The drawing under review shows one solid part. Ordinate dimensions are in mm from its lowest x, y, z. A direction names the side the tool comes from. Round coordinates to 2 decimals unless told otherwise and drop trailing zeros. Order: outer loops, then holes, each group sorted by start corner. A loop starts at its lowest first (then second) coordinate and runs counter-clockwise, first axis right, second up. Notation, with made-up numbers: (28, 73) -> (84, 73) arc R8 cw to (84, 78) -> close; hole circle Ø10 at (-28.5, 75). An arc over 180 degrees is marked (long way). Put each result on its own line as item: value. Start each with the question number.
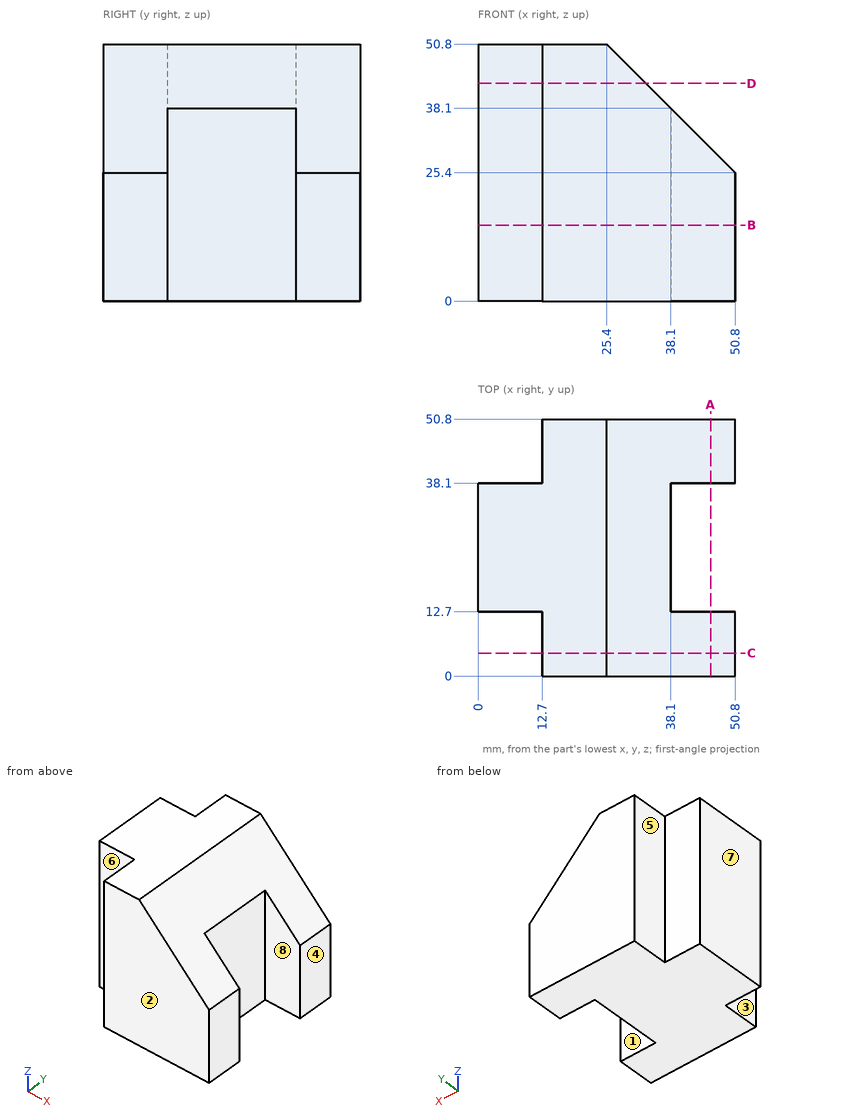
Item 1: Consider section C-C, the plane y = 4.5. Write out the cut boundary in (x, z).
Item 2: Consider section B-B, the plane z = 15. Write out the cut boundary in (x, y).
Item 3: Tool access review of the marked faces 1, 2, 3, 4 and 5: name each direction out of +Z, -Z, +X, -X, +Y, -Y from which nothing blocks a thin tool from reaching the whole face with its end or side.
Item 4: Mouldability with a two-part tool opening along Y and no side actions: class the marked faces 6, 7 and 8 as +Y half, -Y half, draft (parallel to the pull), parting line (faces both ways), or undercut.
Item 5: For L1, parallel to Y at x = 39, z = 30; L2, parallel to Y at x = 11.5, z = 11; L3, parallel to X at y = 29.5, z = 14.5, list the stretches that pass through material, from the lowest coordinate up.
Item 6: Consider section A-A, the plane x = 46. Write out the cut boundary in (y, z), plus the area to 3 significant figures.
Item 7: Insertion check: pin 1 Ø4 at (x, z) = (5.5, 17.5) entering from +Y; pin 2 Ø8 at (x, y) = (30.5, 23.5) entering from +Z; pin 3 Ø14 at (x, z) = (5, 33.5) entering from -Y. Each pin has a flat end and moves straight along its axis. Give the tip position at first contact, or say it passes through.
Item 8: Consider section D-D, the plane z = 43. Write out the cut boundary in (x, y).
Evaluation:
1. outline: (12.7, 0) -> (50.8, 0) -> (50.8, 25.4) -> (25.4, 50.8) -> (12.7, 50.8) -> close
2. outline: (0, 12.7) -> (12.7, 12.7) -> (12.7, 0) -> (50.8, 0) -> (50.8, 12.7) -> (38.1, 12.7) -> (38.1, 38.1) -> (50.8, 38.1) -> (50.8, 50.8) -> (12.7, 50.8) -> (12.7, 38.1) -> (0, 38.1) -> close
3. face 1: +Z, -Z, +X
3. face 2: +Z, -Z, +X, -X, -Y
3. face 3: +Z, -Z, -X, -Y
3. face 4: +Z, -Z, +X, +Y, -Y
3. face 5: +Z, -Z, -X, +Y
4. face 6: -Y half
4. face 7: draft
4. face 8: undercut
5. L1: y = 0 to 12.7, 38.1 to 50.8
5. L2: y = 12.7 to 38.1
5. L3: x = 0 to 38.1
6. outline: (0, 0) -> (12.7, 0) -> (12.7, 30.2) -> (0, 30.2) -> close; (38.1, 0) -> (50.8, 0) -> (50.8, 30.2) -> (38.1, 30.2) -> close
6. area: 767 mm^2
7. pin 1: stops at y = 38.1
7. pin 2: stops at z = 49.7
7. pin 3: stops at y = 12.7
8. outline: (0, 12.7) -> (12.7, 12.7) -> (12.7, 0) -> (33.2, 0) -> (33.2, 50.8) -> (12.7, 50.8) -> (12.7, 38.1) -> (0, 38.1) -> close
